Read the model definition and answer for the solid it produces. Units are mm, in the model's axes. A direction names the side the tool comes from. Give positions to 0.01 mm unless a question says otherwise; leave off trailing zeros. Write each loop counter-clockwise with the first axis right and the second up, starting at its lowest first coordinate (ties: lowest second). Pieces come first, ordered by that corner, then holes. Notation, with made-up numbers: (24, 59) -> (61, 59) arc R28 cw to (61, 96) -> close; hole circle Ø1 at (1, 74.5). An arc over 180 degrees is marked (long way). Answer as CSV lines item,"result". Start each with the question number.
1. For a pull along Y with two mould halves and no side action, classify faces 1 (the flat face through (27, -6.7, 41.5)), 2 (the flat face through (0, 0, 0)), 3 (the flat face through (0, 15, 23)) as pulls with the +Y half, pulls with the -Y half, needs draft (parallel to the pull), parting line crosses it, or undercut.
2. Find the intervals of material crossed by line 1 (Y direction, x = -19.5, z = 22.5); line 2 (X direction, y = 0.25, z = 19.5); line 3 (Z direction, x = -30.8, y = -9.25), in increasing order.
3. The part is cut by section A-A, the plane x = 4. Determine the outline of the cut face in (y, z).
4. A tool of negligible diameter and unlimited length cuts with its end or side. For faces 4 (the flat face through (-32, -9, 43)), 5 (the flat face through (30, -5.5, 42)), 6 (the cylindrical face through (5.386, -14.014, 4.925)), from which of +Z, -Z, +X, -X, +Y, -Y can it reach the whole face along a straight path? Write none if from no direction.
5. The part is cut by section B-B, the plane z = 42.25. Determine the outline of the cut face in (x, y).
6. The part is cut by section C-C, the plane x = 13.5. Determine the outline of the cut face in (y, z), and give its area (3 significant figures).
7. The part is cut by section D-D, the plane y = -9.25. Determine the outline of the cut face in (x, z).
from build123d import *

# Parameters (mm, degrees)
F0_W     = 68
F0_H     = 30
F0_W_2   = 64
F0_H_2   = 26
F1_DEPTH = 46
F2_DEPTH = 2
F3_R     = 1.5
F4_DEPTH = 3
F6_DEPTH = 5
F8_DEPTH = 5


with BuildPart() as f1:
    # F0 (on Top) → F1 (new body)
    with BuildSketch(Plane.XY):
        Rectangle(F0_W, F0_H)
        Rectangle(F0_W_2, F0_H_2, mode=Mode.SUBTRACT)
    extrude(amount=F1_DEPTH)

    # F0 (on Top) → F2 (join)
    with BuildSketch(Plane.XY):
        Rectangle(F0_W, F0_H)
        Rectangle(F0_W_2, F0_H_2, mode=Mode.SUBTRACT)
        Rectangle(F0_W_2, F0_H_2)
    extrude(amount=F2_DEPTH)

    # F3 (on face) → F4 (cut)
    with BuildSketch(Plane.XZ.offset(15)):
        with Locations((4, 5.5)):
            Circle(F3_R)
    extrude(amount=-F4_DEPTH, mode=Mode.SUBTRACT)

    # F5 (on face) → F6 (join)
    with BuildSketch(Plane.YZ.offset(-32)):
        with BuildLine():
            Line((-10.5, 46), (-13, 46))
            Line((-13, 46), (-13, 38.5))
            Line((-13, 38.5), (-10.5, 38.5))
            Line((-10.5, 38.5), (-8, 38.5))
            Line((-8, 38.5), (-5.5, 38.5))
            Line((-5.5, 38.5), (-5.5, 46))
            Line((-5.5, 46), (-8, 46))
            Line((-8, 46), (-8, 44.415064))
            ThreePointArc((-8, 44.415064), (-9.25, 39.75), (-10.5, 44.415064))
            Line((-10.5, 44.415064), (-10.5, 46))
        make_face()
    extrude(amount=F6_DEPTH)

    # F7 (on face) → F8 (join)
    with BuildSketch(Plane(origin=(32, 0, 0), x_dir=(0, -1, 0), z_dir=(-1, 0, 0))):
        with BuildLine():
            Line((13, 38.5), (13, 46))
            Line((13, 46), (10.5, 46))
            Line((10.5, 46), (10.5, 44.415064))
            ThreePointArc((10.5, 44.415064), (9.25, 39.75), (8, 44.415064))
            Line((8, 44.415064), (8, 46))
            Line((8, 46), (5.5, 46))
            Line((5.5, 46), (5.5, 38.5))
            Line((5.5, 38.5), (8, 38.5))
            Line((8, 38.5), (10.5, 38.5))
            Line((10.5, 38.5), (13, 38.5))
        make_face()
    extrude(amount=F8_DEPTH)


solid = f1.part
Results found:
1,face 1,"undercut"
1,face 2,"needs draft"
1,face 3,"pulls with the +Y half"
2,line 1,"y = -15 to -13, 13 to 15"
2,line 2,"x = -34 to -32, 32 to 34"
2,line 3,"z = 0 to 2, 38.5 to 39.75"
3,outline,"(-15, 0) -> (15, 0) -> (15, 46) -> (13, 46) -> (13, 2) -> (-13, 2) -> (-13, 4) -> (-15, 4) -> close; (-15, 7) -> (-13, 7) -> (-13, 46) -> (-15, 46) -> close"
4,face 4,"none"
4,face 5,"+Z"
4,face 6,"-Y"
5,outline,"(-34, -15) -> (34, -15) -> (34, 15) -> (-34, 15) -> close; hole (-32, -11.75) -> (-27, -11.75) -> (-27, -13) -> (27, -13) -> (27, -11.75) -> (32, -11.75) -> (32, -6.75) -> (27, -6.75) -> (27, -5.5) -> (32, -5.5) -> (32, 13) -> (-32, 13) -> (-32, -5.5) -> (-27, -5.5) -> (-27, -6.75) -> (-32, -6.75) -> close"
6,outline,"(-15, 0) -> (15, 0) -> (15, 46) -> (13, 46) -> (13, 2) -> (-13, 2) -> (-13, 46) -> (-15, 46) -> close"
6,area,"236 mm²"
7,outline,"(-34, 0) -> (34, 0) -> (34, 46) -> (32, 46) -> (32, 39.75) -> (27, 39.75) -> (27, 38.5) -> (32, 38.5) -> (32, 2) -> (-32, 2) -> (-32, 38.5) -> (-27, 38.5) -> (-27, 39.75) -> (-32, 39.75) -> (-32, 46) -> (-34, 46) -> close"
